from build123d import *

# Parameters (mm, degrees)
BOSS_EXTRUDE1_DEPTH             = 0.5
BOSS_EXTRUDE1_DRAFT             = 21.801409486
BOSS_EXTRUDE2_DEPTH             = 1.5
CUT_EXTRUDE1_DEPTH              = 1
SKETCH4_W                       = 5
SKETCH4_H                       = 4
CUT_EXTRUDE2_DEPTH              = 0.5
SKETCH5_W                       = 0.8
SKETCH5_H                       = 9.4
BOSS_EXTRUDE3_DEPTH             = 1
SKETCH6_W                       = 5
SKETCH6_H                       = 4
CUT_EXTRUDE3_DEPTH              = 0.5
SKETCH7_W                       = 5
SKETCH7_H                       = 4
CUT_EXTRUDE4_DEPTH              = 0.5
SKETCH8_W                       = 0.8
SKETCH8_H                       = 9.4
BOSS_EXTRUDE4_DEPTH             = 1
SKETCH9_W                       = 5
SKETCH9_H                       = 4
CUT_EXTRUDE5_DEPTH              = 0.5
BOSS_EXTRUDE5_DEPTH             = 1
BOSS_EXTRUDE6_DEPTH             = 1
DRAFT1_ANGLE                    = -8.423132134
SKETCH12_W                      = 2.5
SKETCH12_H                      = 1
SKETCH13_W                      = 2.5
SKETCH13_H                      = 1
SKETCH14_W                      = 2.5
SKETCH14_H                      = 1
SKETCH15_W                      = 2.5
SKETCH15_H                      = 1
SKETCH16_W                      = 2.5
SKETCH16_H                      = 1
SKETCH17_W                      = 2.5
SKETCH17_H                      = 1
SKETCH18_W                      = 2.5
SKETCH18_H                      = 1
SKETCH19_W                      = 2.5
SKETCH19_H                      = 1
SKETCH20_W                      = 2.5
SKETCH20_H                      = 1
SKETCH21_W                      = 2.5
SKETCH21_H                      = 1
SKETCH22_W                      = 2.5
SKETCH22_H                      = 1
SKETCH23_W                      = 2.5
SKETCH23_H                      = 1
SKETCH24_W                      = 2.5
SKETCH24_H                      = 1
SKETCH25_W                      = 2.5
SKETCH25_H                      = 1
M3X0_5_TAPPED_HOLE1_D           = 1.6
M3X0_5_TAPPED_HOLE1_CBORE_D     = 3
M3X0_5_TAPPED_HOLE1_CBORE_DEPTH = 1
F_6_0_6_DIAMETER_HOLE1_D        = 6
F_6_0_6_DIAMETER_HOLE1_DEPTH    = 0.5
FILLET2_R                       = 0.1


with BuildPart() as part:
    # Sketch1 → Boss-Extrude1 (with draft: the straight prism first)
    with BuildSketch(Plane(origin=(0, 2, 0), x_dir=(1, 0, 0), z_dir=(0, 1, 0))):
        Polygon((24.217912597, -38.196520554), (31.8, -0.078793123), (31.8, 28.981304325), (19.4, 28.981304325), (19.4, 20.981304325), (-0.2, 20.981304325), (-0.2, 28.981304325), (-20.6, 28.981304325), (-20.6, -79.418695675), (-0.2, -79.418695675), (-0.2, -25.874898862), (13.618871878, -27.92119344), (12.05617512, -35.777400561), align=None)
    extrude(amount=-BOSS_EXTRUDE1_DEPTH)
    # Boss-Extrude1: the draft: its side faces are tilted about the plane it starts from
    boss_extrude1_sides = [part.faces().sort_by_distance(p)[0] for p in [
        (28.008956299, 1.75, 19.137656838),
        (31.8, 1.75, -14.451255601),
        (25.6, 1.75, -28.981304325),
        (19.4, 1.75, -24.981304325),
        (9.6, 1.75, -20.981304325),
        (-0.2, 1.75, -24.981304325),
        (-10.4, 1.75, -28.981304325),
        (-20.6, 1.75, 25.218695675),
        (-10.4, 1.75, 79.418695675),
        (-0.2, 1.75, 52.646797268),
        (6.709435939, 1.75, 26.898046151),
        (12.837523499, 1.75, 31.849297001),
        (18.137043859, 1.75, 36.986960558),
    ]]
    draft(boss_extrude1_sides, Plane(origin=(0, 2, 0), x_dir=(1, 0, 0), z_dir=(0, 1, 0)), BOSS_EXTRUDE1_DRAFT)

    # Sketch2 → Boss-Extrude2 (add)
    with BuildSketch(Plane.XZ.offset(-1.5)):
        Polygon((32, -29.181304325), (19.2, -29.181304325), (19.2, -21.181304325), (0, -21.181304325), (0, -29.181304325), (-20.8, -29.181304325), (-20.8, 79.618695675), (0, 79.618695675), (0, 26.106695675), (13.381722576, 28.08825731), (11.821, 35.934539553), (24.375051589, 38.431695675), (32, 0.098491403), align=None)
    extrude(amount=BOSS_EXTRUDE2_DEPTH)

    # Sketch3 → Cut-Extrude1 (cut)
    with BuildSketch(Plane(origin=(0, 2, 0), x_dir=(-1, 0, 0), z_dir=(0, 1, 0))):
        Polygon((19.8, -28.181304325), (19.8, 78.618695675), (1, 78.618695675), (1, 24.947711614), (-15.026007114, 24.947711614), (-12.996875602, 35.148844594), (-23.589356631, 37.255820072), (-31, 0), (-31, -28.181304325), (-20.2, -28.181304325), (-20.2, -20.181304325), (1, -20.181304325), (1, -28.181304325), align=None)
    extrude(amount=-CUT_EXTRUDE1_DEPTH, mode=Mode.SUBTRACT)

    # Sketch4 → Cut-Extrude2 (cut)
    with BuildSketch(Plane(origin=(0, 1, 0), x_dir=(-1, 0, 0), z_dir=(0, 1, 0))):
        with Locations((4.4, 8.218695675)):
            Rectangle(SKETCH4_W, SKETCH4_H)
    extrude(amount=-CUT_EXTRUDE2_DEPTH, mode=Mode.SUBTRACT)

    # Sketch5 → Boss-Extrude3 (add)
    with BuildSketch(Plane(origin=(0, 1, 0), x_dir=(-1, 0, 0), z_dir=(0, 1, 0))):
        with Locations((6, 1.518695675)):
            Rectangle(SKETCH5_W, SKETCH5_H)
    extrude(amount=BOSS_EXTRUDE3_DEPTH)

    # Sketch6 → Cut-Extrude3 (cut)
    with BuildSketch(Plane(origin=(0, 1, 0), x_dir=(-1, 0, 0), z_dir=(0, 1, 0))):
        with Locations((4.4, -5.181304325)):
            Rectangle(SKETCH6_W, SKETCH6_H)
    extrude(amount=-CUT_EXTRUDE3_DEPTH, mode=Mode.SUBTRACT)

    # Sketch7 → Cut-Extrude4 (cut)
    with BuildSketch(Plane(origin=(0, 1, 0), x_dir=(-1, 0, 0), z_dir=(0, 1, 0))):
        with Locations((14.4, 8.218695675)):
            Rectangle(SKETCH7_W, SKETCH7_H)
    extrude(amount=-CUT_EXTRUDE4_DEPTH, mode=Mode.SUBTRACT)

    # Sketch8 → Boss-Extrude4 (add)
    with BuildSketch(Plane(origin=(0, 1, 0), x_dir=(-1, 0, 0), z_dir=(0, 1, 0))):
        with Locations((12.8, 1.518695675)):
            Rectangle(SKETCH8_W, SKETCH8_H)
    extrude(amount=BOSS_EXTRUDE4_DEPTH)

    # Sketch9 → Cut-Extrude5 (cut)
    with BuildSketch(Plane(origin=(0, 1, 0), x_dir=(-1, 0, 0), z_dir=(0, 1, 0))):
        with Locations((14.4, -5.181304325)):
            Rectangle(SKETCH9_W, SKETCH9_H)
    extrude(amount=-CUT_EXTRUDE5_DEPTH, mode=Mode.SUBTRACT)

    # Sketch10 → Boss-Extrude5 (add)
    with BuildSketch(Plane(origin=(0, 1, 0), x_dir=(-1, 0, 0), z_dir=(0, 1, 0))):
        with BuildLine():
            Line((10.8, 78.618695675), (10.8, 31.618695675))
            ThreePointArc((10.8, 31.618695675), (10.4, 31.218695675), (10, 31.618695675))
            Line((10, 31.618695675), (10, 78.618695675))
            Line((10, 78.618695675), (10.8, 78.618695675))
        make_face()
    extrude(amount=BOSS_EXTRUDE5_DEPTH)

    # Sketch11 → Boss-Extrude6 (add)
    with BuildSketch(Plane(origin=(0, 1, 0), x_dir=(-1, 0, 0), z_dir=(0, 1, 0))):
        with BuildLine():
            Line((-1.2, 0.818695675), (-23.8, 0.818695675))
            ThreePointArc((-23.8, 0.818695675), (-24.2, 1.218695675), (-23.8, 1.618695675))
            Line((-23.8, 1.618695675), (-1.2, 1.618695675))
            ThreePointArc((-1.2, 1.618695675), (-0.8, 1.218695675), (-1.2, 0.818695675))
        make_face()
    extrude(amount=BOSS_EXTRUDE6_DEPTH)

    # Draft1
    draft1_faces = [part.faces().sort_by_distance(p)[0] for p in [
        (7.013003557, 1.5, 24.947711614),
    ]]
    draft(draft1_faces, Plane(origin=(-1, 1, 78.618695675), x_dir=(0, 0, -1), z_dir=(-1, 0, 0)), DRAFT1_ANGLE)

    # Sketch12 → Revolve1 (revolve)
    with BuildSketch(Plane.XY.offset(-6.881304325)):
        with Locations((1.85, 1.5)):
            Rectangle(SKETCH12_W, SKETCH12_H)
    revolve(axis=Axis((0.6, 2, -6.881304325), (0, -1, 0)))

    # Sketch13 → Revolve2 (revolve)
    with BuildSketch(Plane.XY.offset(73.318695675), mode=Mode.PRIVATE) as revolve2_sk:
        with Locations((-14.55, 1.5)):
            Rectangle(SKETCH13_W, SKETCH13_H)
    revolve(revolve2_sk.sketch.rotate(Axis((-15.8, 2, 73.318695675), (0, -1, 0)), 270), axis=Axis((-15.8, 2, 73.318695675), (0, -1, 0)))

    # Sketch14 → Revolve3 (revolve)
    with BuildSketch(Plane.XY.offset(73.318695675), mode=Mode.PRIVATE) as revolve3_sk:
        with Locations((-3.75, 1.5)):
            Rectangle(SKETCH14_W, SKETCH14_H)
    revolve(revolve3_sk.sketch.rotate(Axis((-5, 2, 73.318695675), (0, -1, 0)), 270), axis=Axis((-5, 2, 73.318695675), (0, -1, 0)))

    # Sketch15 → Revolve4 (revolve)
    with BuildSketch(Plane.XY.offset(31.118695675), mode=Mode.PRIVATE) as revolve4_sk:
        with Locations((-14.55, 1.5)):
            Rectangle(SKETCH15_W, SKETCH15_H)
    revolve(revolve4_sk.sketch.rotate(Axis((-15.8, 2, 31.118695675), (0, -1, 0)), 270), axis=Axis((-15.8, 2, 31.118695675), (0, -1, 0)))

    # Sketch16 → Revolve5 (revolve)
    with BuildSketch(Plane.XY.offset(31.118695675), mode=Mode.PRIVATE) as revolve5_sk:
        with Locations((-3.75, 1.5)):
            Rectangle(SKETCH16_W, SKETCH16_H)
    revolve(revolve5_sk.sketch.rotate(Axis((-5, 2, 31.118695675), (0, -1, 0)), 270), axis=Axis((-5, 2, 31.118695675), (0, -1, 0)))

    # Sketch17 → Revolve6 (revolve)
    with BuildSketch(Plane.XY.offset(14.118695675), mode=Mode.PRIVATE) as revolve6_sk:
        with Locations((-14.55, 1.5)):
            Rectangle(SKETCH17_W, SKETCH17_H)
    revolve(revolve6_sk.sketch.rotate(Axis((-15.8, 2, 14.118695675), (0, -1, 0)), 270), axis=Axis((-15.8, 2, 14.118695675), (0, -1, 0)))

    # Sketch18 → Revolve7 (revolve)
    with BuildSketch(Plane.XY.offset(-10.881304325), mode=Mode.PRIVATE) as revolve7_sk:
        with Locations((-14.55, 1.5)):
            Rectangle(SKETCH18_W, SKETCH18_H)
    revolve(revolve7_sk.sketch.rotate(Axis((-15.8, 2, -10.881304325), (0, -1, 0)), 270), axis=Axis((-15.8, 2, -10.881304325), (0, -1, 0)))

    # Sketch19 → Revolve8 (revolve)
    with BuildSketch(Plane.XY.offset(-23.781304325), mode=Mode.PRIVATE) as revolve8_sk:
        with Locations((-14.55, 1.5)):
            Rectangle(SKETCH19_W, SKETCH19_H)
    revolve(revolve8_sk.sketch.rotate(Axis((-15.8, 2, -23.781304325), (0, -1, 0)), 270), axis=Axis((-15.8, 2, -23.781304325), (0, -1, 0)))

    # Sketch20 → Revolve9 (revolve)
    with BuildSketch(Plane.XY.offset(-23.781304325), mode=Mode.PRIVATE) as revolve9_sk:
        with Locations((-3.75, 1.5)):
            Rectangle(SKETCH20_W, SKETCH20_H)
    revolve(revolve9_sk.sketch.rotate(Axis((-5, 2, -23.781304325), (0, -1, 0)), 270), axis=Axis((-5, 2, -23.781304325), (0, -1, 0)))

    # Sketch21 → Revolve10 (revolve)
    with BuildSketch(Plane.XY.offset(-23.781304325)):
        with Locations((26.85, 1.5)):
            Rectangle(SKETCH21_W, SKETCH21_H)
    revolve(axis=Axis((25.6, 2, -23.781304325), (0, -1, 0)))

    # Sketch22 → Revolve11 (revolve)
    with BuildSketch(Plane.XY.offset(-6.881304325), mode=Mode.PRIVATE) as revolve11_sk:
        with Locations((20.95, 1.5)):
            Rectangle(SKETCH22_W, SKETCH22_H)
    revolve(revolve11_sk.sketch.rotate(Axis((19.7, 2, -6.881304325), (0, -1, 0)), 270), axis=Axis((19.7, 2, -6.881304325), (0, -1, 0)))

    # Sketch23 → Revolve12 (revolve)
    with BuildSketch(Plane.XY.offset(10.318695675), mode=Mode.PRIVATE) as revolve12_sk:
        with Locations((20.95, 1.5)):
            Rectangle(SKETCH23_W, SKETCH23_H)
    revolve(revolve12_sk.sketch.rotate(Axis((19.7, 2, 10.318695675), (0, -1, 0)), 270), axis=Axis((19.7, 2, 10.318695675), (0, -1, 0)))

    # Sketch24 → Revolve13 (revolve)
    with BuildSketch(Plane.XY.offset(31.972205419), mode=Mode.PRIVATE) as revolve13_sk:
        with Locations((20.384540675, 1.5)):
            Rectangle(SKETCH24_W, SKETCH24_H)
    revolve(revolve13_sk.sketch.rotate(Axis((19.134540675, 2, 31.972205419), (0, -1, 0)), 270), axis=Axis((19.134540675, 2, 31.972205419), (0, -1, 0)))

    # Sketch25 → Revolve14 (revolve)
    with BuildSketch(Plane.XY.offset(10.318695675)):
        with Locations((1.85, 1.5)):
            Rectangle(SKETCH25_W, SKETCH25_H)
    revolve(axis=Axis((0.6, 2, 10.318695675), (0, -1, 0)))

    # M3x0.5 Tapped Hole1 (through all)
    with Locations(Plane(origin=(0, 0, 0), x_dir=(-1, 0, 0), z_dir=(0, -1, 0))):
        with Locations((15.8, 10.881304325), (5, 23.781304325), (-19.7, 6.881304325), (-19.134540675, -31.972205419), (15.8, -14.118695675), (15.8, -31.118695675), (15.8, -73.318695675), (5, -73.318695675), (5, -31.118695675), (-0.6, -10.318695675), (-19.7, -10.318695675), (-25.6, 23.781304325), (15.8, 23.781304325), (-0.6, 6.881304325)):
            CounterBoreHole(M3X0_5_TAPPED_HOLE1_D / 2, M3X0_5_TAPPED_HOLE1_CBORE_D / 2, M3X0_5_TAPPED_HOLE1_CBORE_DEPTH)

    # Ø6.0 (6) Diameter Hole1
    with Locations(Plane(origin=(0, 1, 0), x_dir=(1, 0, 0), z_dir=(0, 1, 0))):
        with Locations((22, 13.581304325)):
            Hole(F_6_0_6_DIAMETER_HOLE1_D / 2, depth=F_6_0_6_DIAMETER_HOLE1_DEPTH)

    # Fillet2
    fillet2_edges = [part.edges().sort_by_distance(p)[0] for p in [
        (23.1, 2, -23.781304325),
    ]]
    fillet(fillet2_edges, radius=FILLET2_R)


solid = part.part
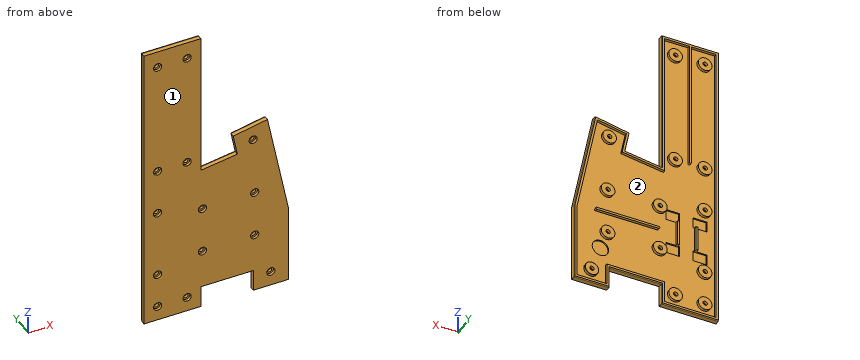
For this review, take the finished solid that the model builds, in its own axes (mm). Face numbers are marked on the shaded views. Round coordinates to 2 decimals unless told otherwise and drop trailing zeros. Write each loop counter-clockwise with the first axis right and the second up, starting at its lowest first coordinate (ties: lowest second). Pieces come first, ordered by that corner, then holes. Notation, with made-up numbers: M 70.25,-17 L 85.25,-17 A16 cw 85.25,12 Z; hole C -19.75,78.5 d10. An arc over 180 degrees is marked long. Write item = value, one per line. Start each with the question number.
(1) Clearance check with flat-ended pins moving along their axes: pin 1 Ø3 at (x, z) = (-15.5, 9) entering from +Y; pin 2 Ø2.5 at (x, z) = (-5, -23.78) entering from -Y. State where each tip first meets the part, or that it passes through.
(2) We need section B-B (x = 8.5). Give the boundary of the cut face in (y, z).
(3) The part is to be moulded in two halves that separate along X. For the marked faces 1 and 2, say which applies: +X half, -X half, draft (parallel to the pull), parting line (faces both ways), or undercut.
(4) We need section C-C (z = -19). Give the boundary of the cut face in (x, y).
(5) We need section A-A (z = 44). Give the boundary of the cut face in (x, y), then the cut area to 3 significant figures.
(6) For line 1 along X through (y, z) = (1.35, 42); line 2 along Z through (x, y) = (-15.8, 0.2); line 3 along X through (y, z) = (1.3, 0), list the stretches that pass through material, from the lowest coordinate up.
Results found:
q1.pin_1 = 1
q1.pin_2 = 1
q2.outline = M 0,-21.18 L 1.5,-21.18 L 2,-20.98 L 2,-20.18 L 1,-20.18 L 1,0.82 L 2,0.82 L 2,1.62 L 1,1.62 L 1,26.35 L 2,26.35 L 2,27.16 L 1.5,27.37 L 0,27.37 Z
q3.face_1 = draft
q3.face_2 = undercut
q4.outline = M -20.8,0 L 32,0 L 32,1.5 L 31.8,2 L 31,2 L 31,1 L -19.8,1 L -19.8,2 L -20.6,2 L -20.8,1.5 Z
q5.outline = M -20.8,0 L 0,0 L 0,1.5 L -0.2,2 L -1,2 L -1,1 L -10,1 L -10,2 L -10.8,2 L -10.8,1 L -19.8,1 L -19.8,2 L -20.6,2 L -20.8,1.5 Z
q5.area = 23.5 mm²
q6.line_1 = -20.8 to -19.8, -10.8 to -10, -1 to 0
q6.line_2 = -29.18 to -25.28, -22.28 to -12.38, -9.38 to 12.62, 15.62 to 29.62, 32.62 to 71.82, 74.82 to 79.62
q6.line_3 = -20.8 to -19.8, -13.2 to -12.4, -6.4 to -5.6, 31 to 32
